from build123d import *

# Parameters (mm, degrees)
SKETCH_1_W          = 25
SKETCH_1_H          = 41
EXTRUDE_1_DEPTH     = 30
FILLET_1_R          = 1
SKETCH_2_R          = 24.95
CUT_EXTRUDE_1_DEPTH = 30


with BuildPart() as part:
    # Эскиз1 → Бобышка-Вытянуть1 (new body)
    with BuildSketch(Plane(origin=(0, 0, 0), x_dir=(1, 0, 0), z_dir=(0, 1, 0))):
        Rectangle(SKETCH_1_W, SKETCH_1_H)
    extrude(amount=EXTRUDE_1_DEPTH)

    # Скругление1
    fillet_1_edges = [part.edges().sort_by_distance(p)[0] for p in [
        (-12.5, 0, 0),
    ]]
    fillet(fillet_1_edges, radius=FILLET_1_R)

    # Эскиз2 → Вырез-Вытянуть1 (cut)
    with BuildSketch(Plane(origin=(0, 30, 0), x_dir=(1, 0, 0), z_dir=(0, 1, 0))):
        with Locations((12.5, 0)):
            Circle(SKETCH_2_R)
    extrude(amount=-CUT_EXTRUDE_1_DEPTH, mode=Mode.SUBTRACT)


solid = part.part
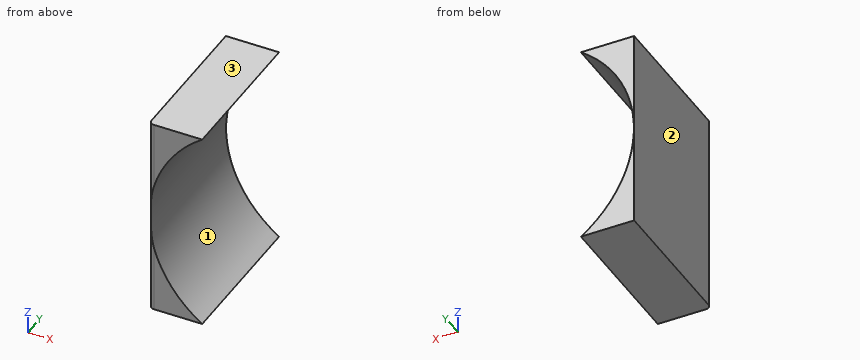
Input: part model. Units: mm. Frame: model coordinates. Face numbers are marked on the shaded views. Coordinates: 2 decimals unless noted, no trailing zeros. Loops run counter-clockwise (first coordinate to the right, second up) from the corner with the lowest first, then second, coordinate; pieces in that order, holes last. Notation, with made-up numbers: (26.25, -8) -> (62.25, -8) arc R11 cw to (62.25, 12) -> close; hole circle Ø4 at (-2.75, 4.5). An arc over 180 degrees is marked (long way). Write each question's results on one line, items separated by ' | '. Start each with the question number.
Q1. Section B-B, the plane y = 18. Return the cut outline in (x, z).
Q2. Section A-A, the plane x = -8. Return the cut outline in (y, z).
Q3. Ray query, line 1 (Z direction, x = -3.5, y = 16); line 2 (Z direction, x = -10, y = 24.5); line 3 (X direction, y = 11, z = -5). Return the intervals inside material, ascending. Write a range as from..to.
Q4. Pull-direction query (Z, two-part tool) for the marked faces 1, 2 and 3; classes: released by +Z, released by -Z, zero draft, split by the parting line, or undercut.
Q5. Section C-C, the plane z = 15.5. Return the cut outline in (x, y), plus the area to 3 significant figures.
Q6. Pin query (flat end, axial travel): pin 1 (8 mm diameter, centred on y = 23.5, z = 6, fed in from +X); pin 2 (10 mm diameter, centred on y = 13, z = -10.5, fed in from +X). Return the tip coordinate at first contact, or that it passes through.
Q7. Section D-D, the plane x = -2.5. Return the cut outline in (y, z).
Found:
1) outline: (-12.5, -20.5) -> (-1.72, -20.5) arc R24.95 cw to (-1.72, 20.5) -> (-12.5, 20.5) -> close
2) outline: (0, -20.5) -> (30, -20.5) -> (30, -14.22) -> (0, -14.22) -> close; (0, 14.22) -> (30, 14.22) -> (30, 20.5) -> (0, 20.5) -> close
3) line 1: -20.5..-19.14, 19.14..20.5 | line 2: -20.5..-10.78, 10.78..20.5 | line 3: -12.5..-11.94
4) face 1: undercut | face 2: zero draft | face 3: released by +Z
5) outline: (-12.5, 1) arc R1 ccw to (-11.5, 0) -> (-7.05, 0) -> (-7.05, 30) -> (-12.5, 30) -> close | area: 163 mm2
6) pin 1: x = -10.36 | pin 2: x = -7.05
7) outline: (0, -20.5) -> (30, -20.5) -> (30, -19.94) -> (0, -19.94) -> close; (0, 19.94) -> (30, 19.94) -> (30, 20.5) -> (0, 20.5) -> close
